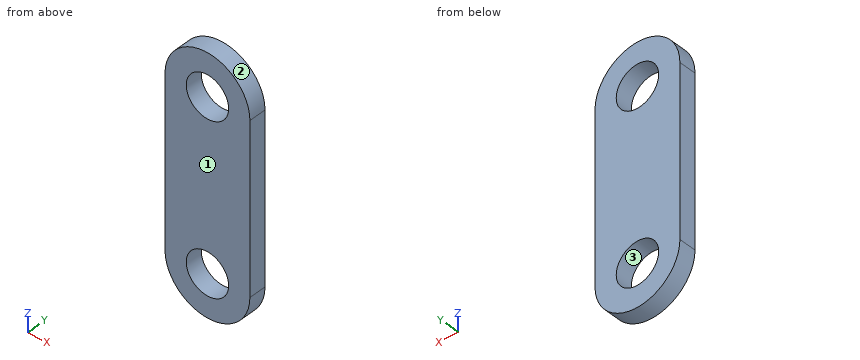
from build123d import *

# Parameters (mm, degrees)
F0_R     = 5
F1_DEPTH = 4


with BuildPart() as f1:
    # F0 (on Front) → F1 (new body)
    with BuildSketch(Plane.XZ):
        with BuildLine():
            ThreePointArc((-10, 0), (0, -10), (10, 0))
            ThreePointArc((10, 0), (0, 10), (-10, 0))
        make_face()
        Circle(F0_R, mode=Mode.SUBTRACT)
        with BuildLine():
            Line((10, -40), (10, 0))
            ThreePointArc((10, 0), (0, -10), (-10, 0))
            Line((-10, 0), (-10, -40))
            ThreePointArc((-10, -40), (0, -30), (10, -40))
        make_face()
        with BuildLine():
            ThreePointArc((-10, -40), (0, -50), (10, -40))
            ThreePointArc((10, -40), (0, -30), (-10, -40))
        make_face()
        with Locations((0, -40)):
            Circle(F0_R, mode=Mode.SUBTRACT)
    extrude(amount=F1_DEPTH)


solid = f1.part
Can you work these out from the model? Positions are in its coordinate system, mm. Face numbers are marked on the shaded views. Round coordinates to 2 decimals unless told otherwise and drop trailing zeros. Loops run counter-clockwise (first coordinate to the right, second up) from the corner with the lowest first, then second, coordinate; pieces in that order, holes last. Notation, with made-up numbers: (36, 71.25) - (61, 71.25) arc R34 cw to (61, 110.25) - close; hole circle Ø9 at (27.25, -21). An arc over 180 degrees is marked (long way). Answer in a Markdown table with one row per item. Add a question column.
Q1. I need wall thicknesses on L1, parallel to Z at x = 0, y = -1.8; L2, parallel to Z at x = 1.5, y = -3.45; L3, parallel to X at y = -2.05, z = -1. Which ranges of each line are inside material? Lowest first, please.
Q2. I want a section at A-A on x = 0. List the corners of the cut face in (y, z) for me.
Q3. I want a section at C-C on x = -8.5. List the corners of the cut face in (y, z) for me.
Q4. We'd pull the mould along Z, two halves only. Please class the marked faces 1, 2 and 3: pulls with the +Z half, pulls with the -Z half, needs draft (parallel to the pull), parting line crosses it, or undercut.
Q5. I want a section at B-B on y = -3.2. List the corners of the cut face in (x, z) for me, and give its area (3 significant figures).
Q6. For pin 1 Ø1 at (x, y) = (-3, -3.5) entering from -Z; pin 2 Ø1 at (x, y) = (-1.5, -1.5) entering from +Z, each with a flat end and sliding along its axis, tell me the tip position at first contact or that it passes through.
A:
| question | item | result |
|---|---|---|
| 1 | L1 | -50 to -45, -35 to -5, 5 to 10 |
| 1 | L2 | -49.89 to -44.77, -35.23 to -4.77, 4.77 to 9.89 |
| 1 | L3 | -10 to -4.9, 4.9 to 10 |
| 2 | outline | (-4, -50) - (0, -50) - (0, -45) - (-4, -45) - close; (-4, -35) - (0, -35) - (0, -5) - (-4, -5) - close; (-4, 5) - (0, 5) - (0, 10) - (-4, 10) - close |
| 3 | outline | (-4, -45.27) - (0, -45.27) - (0, 5.27) - (-4, 5.27) - close |
| 4 | face 1 | needs draft |
| 4 | face 2 | pulls with the +Z half |
| 4 | face 3 | undercut |
| 5 | outline | (-10, -40) arc R10 ccw to (10, -40) - (10, 0) arc R10 ccw to (-10, 0) - close; hole circle Ø10 at (0, -40); hole circle Ø10 at (0, 0) |
| 5 | area | 957 mm^2 |
| 6 | pin 1 | z = -49.68 |
| 6 | pin 2 | z = 9.95 |
